```python
from build123d import *

# Parameters (mm, degrees)
CROQUIS3_W              = 12.5
CROQUIS3_H              = 12.5
SALIENTE_EXTRUIR1_DEPTH = 7.35
CROQUIS4_W              = 10.5
CROQUIS4_H              = 6.75
SALIENTE_EXTRUIR2_DEPTH = 3
CROQUIS5_W              = 0.5
CROQUIS5_H              = 4.284238858
SALIENTE_EXTRUIR3_DEPTH = 7


with BuildPart() as part:
    # Croquis2 → Revolución1 (revolve)
    with BuildSketch(Plane.XY, mode=Mode.PRIVATE) as revoluci_n1_sk:
        with BuildLine():
            Line((0, 3.679432079), (-8.659361316, 3.679432079))
            ThreePointArc((-8.659361316, 3.679432079), (-11.14229204, 2.791903832), (-12.5, 0.531532079))
            Line((-12.5, 0.531532079), (-13.888119122, 0.531532079))
            ThreePointArc((-13.888119122, 0.531532079), (-15.961182203, -0.355908417), (-16.75, -2.468467921))
            Line((-16.75, -2.468467921), (-14.75, -2.468467921))
            Line((-14.75, -2.468467921), (-14.75, -14.670168674))
            ThreePointArc((-14.75, -14.670168674), (-13.930397127, -16.648865047), (-11.951700754, -17.468467921))
            Line((-11.951700754, -17.468467921), (0, -17.468467921))
            Line((0, -17.468467921), (0, 3.679432079))
        make_face()
    revolve(revoluci_n1_sk.sketch.rotate(Axis((0, 0, 0), (0, 1, 0)), 270), axis=Axis((0, 0, 0), (0, 1, 0)))

    # Croquis3 → Saliente-Extruir1 (add)
    with BuildSketch(Plane.XZ.offset(17.468467921)):
        Rectangle(CROQUIS3_W, CROQUIS3_H)
    extrude(amount=SALIENTE_EXTRUIR1_DEPTH)

    # Croquis4 → Saliente-Extruir2 (add)
    with BuildSketch(Plane(origin=(0, -24.818467921, 0), x_dir=(-1, 0, 0), z_dir=(0, -1, 0))):
        with Locations((0, 2.375)):
            Rectangle(CROQUIS4_W, CROQUIS4_H)
    extrude(amount=SALIENTE_EXTRUIR2_DEPTH)

    # Croquis5 → Saliente-Extruir3 (add)
    with BuildSketch(Plane.XZ.offset(27.818467921)):
        with Locations((-2.79, -2.875)):
            Rectangle(CROQUIS5_W, CROQUIS5_H)
    saliente_extruir3 = extrude(amount=SALIENTE_EXTRUIR3_DEPTH)

    # Simetría1: Saliente-Extruir3 across plane
    add(saliente_extruir3.mirror(Plane(origin=(0, 0, 0), x_dir=(0, 0, 1), z_dir=(1, 0, 0))))


solid = part.part
```
Could you check a few things on this model? Use its own coordinates, in mm. A direction names the side the tool comes from. Coordinates: 2 decimals unless noted, no trailing zeros. Write each loop counter-clockwise with the first axis right and the second up, starting at its lowest first coordinate (ties: lowest second). Pieces come first, ordered by that corner, then holes. Notation, with made-up numbers: (39.5, 53.5) - (72.5, 53.5) arc R23 ccw to (72.5, 65.5) - close; hole circle Ø9 at (-38, -3). An arc over 180 degrees is marked (long way). Use a Markdown table: item, result.
Q1. Which directions (+Z, -Z, +X, -X, +Y, -Y) give clear straight access to the entire face, cutting with the end or side of a thin tool? Please do faces 4 (the flat face through (2.54, -31, -3)), 5 (the flat face through (-6.25, -21, 0)), 6 (the flat face through (-7.3, 0.532, -10.4)).
Geometry check:
| item | result |
|---|---|
| face 4 | +Z, -Z, -Y |
| face 5 | +Z, -Z, -X, -Y |
| face 6 | +Y |
Q2. I'm going to push flat-ended pins straight in: pin 1 Ø2.5 at (y, z) = (-26, -1) entering from +X; pin 2 Ø10 at (y, z) = (-21.5, -11.5) entering from -X; pin 3 Ø6 at (x, y) = (1.5, -19.5) entering from -Z; pin 4 Ø8 at (y, z) = (-29, 10) entering from +X. Where does each tip first touch, or does it pass through?
Geometry check:
| item | result |
|---|---|
| pin 1 | stops at x = 6.25 |
| pin 2 | stops at x = -9.77 |
| pin 3 | stops at z = -14 |
| pin 4 | passes through |
Q3. Imagine slicing it at B-B (z = 0). List the corners of the cut face in (x, y) for me.
Geometry check:
| item | result |
|---|---|
| outline | (-16.75, -2.47) - (-14.75, -2.47) - (-14.75, -14.67) arc R2.8 ccw to (-11.95, -17.47) - (-6.25, -17.47) - (-6.25, -24.82) - (-5.25, -24.82) - (-5.25, -27.82) - (5.25, -27.82) - (5.25, -24.82) - (6.25, -24.82) - (6.25, -17.47) - (11.95, -17.47) arc R2.8 ccw to (14.75, -14.67) - (14.75, -2.47) - (16.75, -2.47) arc R2.87 ccw to (13.89, 0.53) - (12.5, 0.53) arc R3.92 ccw to (8.66, 3.68) - (-8.66, 3.68) arc R3.92 ccw to (-12.5, 0.53) - (-13.89, 0.53) arc R2.87 ccw to start |
Q4. Imagine slicing it at A-A (x = 0). List the corners of the cut face in (y, z) for me.
Geometry check:
| item | result |
|---|---|
| outline | (-27.82, -5.75) - (-24.82, -5.75) - (-24.82, -6.25) - (-17.47, -6.25) - (-17.47, -11.95) arc R2.8 ccw to (-14.67, -14.75) - (-2.47, -14.75) - (-2.47, -16.75) arc R2.87 ccw to (0.53, -13.89) - (0.53, -12.5) arc R3.92 ccw to (3.68, -8.66) - (3.68, 8.66) arc R3.92 ccw to (0.53, 12.5) - (0.53, 13.89) arc R2.87 ccw to (-2.47, 16.75) - (-2.47, 14.75) - (-14.67, 14.75) arc R2.8 ccw to (-17.47, 11.95) - (-17.47, 6.25) - (-24.82, 6.25) - (-24.82, 1) - (-27.82, 1) - close |
Q5. Thinking about a two-plate mould opening in X: for faces 1 (the flat face through (0, -27.818, -2)), 2 (the flat face through (0, -26, 1)), 3 (the flat face through (5.25, -26, -2)), which applies, +X half, -X half, draft (parallel to the pull), parting line (faces both ways), or undercut?
Geometry check:
| item | result |
|---|---|
| face 1 | undercut |
| face 2 | draft |
| face 3 | +X half |
Q6. Imagine slicing it at D-D (y = -9). List the corners of the cut face in (x, z) for me.
Geometry check:
| item | result |
|---|---|
| outline | circle Ø29.5 at (0, 0) |
Q7. Please list where these lines run through material, in increasing order: L1, parallel to Z at x = 0, y = -20.5; L2, parallel to Y at x = -7, z = -1.5.
Geometry check:
| item | result |
|---|---|
| L1 | z = -6.25 to 6.25 |
| L2 | y = -17.47 to 3.68 |
Q8. Imagine slicing it at C-C (y = -23). List the corners of the cut face in (x, z) for me.
Geometry check:
| item | result |
|---|---|
| outline | (-6.25, -6.25) - (6.25, -6.25) - (6.25, 6.25) - (-6.25, 6.25) - close |
